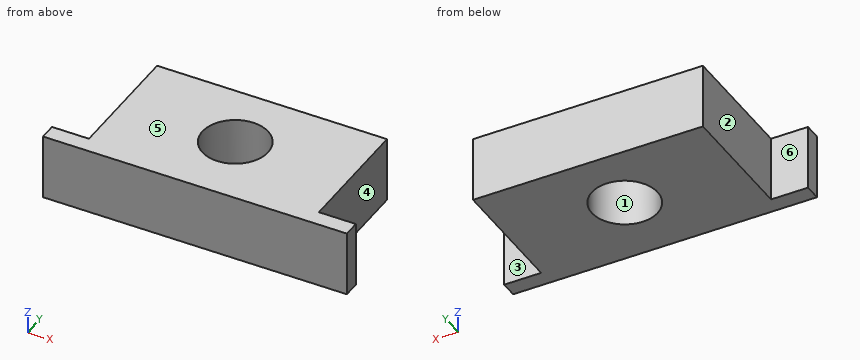
from build123d import *

# Parameters (mm, degrees)
SKETCH1_W           = 58.7502
SKETCH1_H           = 12.7
BOSS_EXTRUDE1_DEPTH = 3.175
SKETCH2_W           = 44.45
SKETCH2_H           = 12.7
BOSS_EXTRUDE2_DEPTH = 24.13
SKETCH3_R           = 6.35
CUT_EXTRUDE1_DEPTH  = 24.13


with BuildPart() as part:
    # Sketch1 → Boss-Extrude1 (new body)
    with BuildSketch(Plane(origin=(0, 0, 0), x_dir=(1, 0, 0), z_dir=(0, 1, 0))):
        with Locations((29.3751, 6.35)):
            Rectangle(SKETCH1_W, SKETCH1_H)
    extrude(amount=BOSS_EXTRUDE1_DEPTH)

    # Sketch2 → Boss-Extrude2 (add)
    with BuildSketch(Plane(origin=(0, 3.175, 0), x_dir=(1, 0, 0), z_dir=(0, 1, 0))):
        with Locations((29.3751, 6.35)):
            Rectangle(SKETCH2_W, SKETCH2_H)
    extrude(amount=BOSS_EXTRUDE2_DEPTH)

    # Sketch3 → Cut-Extrude1 (cut)
    with BuildSketch(Plane.XY):
        with Locations((29.3751, 14.2748)):
            Circle(SKETCH3_R)
    extrude(amount=-CUT_EXTRUDE1_DEPTH, mode=Mode.SUBTRACT)


solid = part.part
Can you work these out from the model? Positions are in its coordinate system, mm. Face numbers are marked on the shaded views. A direction names the side the tool comes from. Round coordinates to 2 decimals unless told otherwise and drop trailing zeros. Order: outer loops, then holes, each group sorted by start corner. A loop starts at its lowest first (then second) coordinate and runs counter-clockwise, first axis right, second up. Notation, with made-up numbers: (19, 5.5) -> (34, 5.5) arc R26 cw to (34, 42.5) -> close; hole circle Ø2 at (-26, 80). An arc over 180 degrees is marked (long way). Write each question's results on one line, items separated by ' | '. Start each with the question number.
Item 1: Thinking about a two-plate mould opening in X: for the marked faces 1, 2 and 3, which applies, +X half, -X half, draft (parallel to the pull), parting line (faces both ways), or undercut?
Item 2: Which directions (+Z, -Z, +X, -X, +Y, -Y) give clear straight access to the entire face, cutting with the end or side of a thin tool? Please do the marked faces 4, 5 and 6.
Item 3: If we section it at C-C, the plane z = -2: Write out the boundary of the cut face in (x, y) (3 decimals).
Item 4: Will these pins go through, and if not, where does the flat tip stop? pin 1 (1.5 mm diameter, centred on y = 11, z = -8, fed in from +X); pin 2 (2 mm diameter, centred on x = 2.5, z = -3.5, fed in from +Y) (3 decimals); pin 3 (4 mm diameter, centred on y = 18.5, z = -8.5, fed in from -X).
Item 5: If we section it at B-B, the plane x = 24.5: Write out the boundary of the cut face in (y, z) (3 decimals).
Item 6: If we section it at A-A, the plane y = 19.75: Write out the boundary of the cut face in (x, z), then the cut area to 3 significant figures.
Item 7: Please list where these lines run through material, in increasing order: L1, parallel to X at y = 22, z = -2.5; L2, parallel to X at y = 10.25, z = -2.5; L3, parallel to X at y = 9, z = -8.75.
Item 8: If we section it at D-D, the plane x = 54.5: Write out the boundary of the cut face in (y, z) (3 decimals).
Results:
1) face 1: undercut | face 2: -X half | face 3: draft
2) face 4: +Z, -Z, +X, +Y | face 5: +Z, +X, -X, +Y, -Y | face 6: +Z, -Z, -X, +Y
3) outline: (0, 0) -> (58.75, 0) -> (58.75, 3.175) -> (51.6, 3.175) -> (51.6, 27.305) -> (7.15, 27.305) -> (7.15, 3.175) -> (0, 3.175) -> close; hole circle Ø12.7 at (29.375, 14.275)
4) pin 1: stops at x = 51.6 | pin 2: stops at y = 3.175 | pin 3: stops at x = 7.15
5) outline: (0, -12.7) -> (10.206, -12.7) -> (10.206, 0) -> (0, 0) -> close; (18.344, -12.7) -> (27.305, -12.7) -> (27.305, 0) -> (18.344, 0) -> close
6) outline: (7.15, -12.7) -> (26.16, -12.7) -> (26.16, 0) -> (7.15, 0) -> close; (32.59, -12.7) -> (51.6, -12.7) -> (51.6, 0) -> (32.59, 0) -> close | area: 483 mm2
7) L1: x = 7.15 to 51.6 | L2: x = 7.15 to 24.46, 34.29 to 51.6 | L3: x = 7.15 to 25.84, 32.91 to 51.6
8) outline: (0, -12.7) -> (3.175, -12.7) -> (3.175, 0) -> (0, 0) -> close
